Design review of the part built by this model. Coordinates are the model's own, in mm. A direction names the side the tool comes from. Give positions to 0.01 mm unless a question says otherwise; leave off trailing zeros. Write each loop counter-clockwise with the first axis right and the second up, starting at its lowest first coordinate (ties: lowest second). Pieces come first, ordered by that corner, then holes. Notation, with made-up numbers: (11, 12.5) - (63, 12.5) arc R14 ccw to (63, 36.5) - close; hole circle Ø5 at (81.25, -32). An arc over 180 degrees is marked (long way). Use a Markdown table: item, result. Add a question column.
```python
from build123d import *

# Parameters (mm, degrees)
F1_DEPTH = 2.1
F3_DEPTH = 1.8
F5_DEPTH = 8
F7_DEPTH = 1.016


with BuildPart() as f1:
    # F0 (on Top) → F1 (new body)
    with BuildSketch(Plane.XY):
        Polygon((61.593626, -18.5), (61.593626, 18.5), (-25.406374, 18.5), (-25.406374, 30.5), (-47.352125, 0), (-25.406374, -30.5), (-25.406374, -18.5), align=None)
    extrude(amount=F1_DEPTH)

    # F2 (on face) → F3 (join)
    with BuildSketch(Plane.XY.offset(2.1)):
        Polygon((59.493628, 16.400002), (-27.506373, 16.400002), (-27.506373, 23.985889), (-44.765007, 0), (-27.506373, -23.985889), (-27.506373, -16.400002), (59.493628, -16.400002), align=None)
        Polygon((-29.606375, 17.471772), (-29.606375, 14.3), (57.393626, 14.3), (57.393626, -14.3), (-29.606375, -14.3), (-29.606375, -17.471772), (-42.177888, 0), align=None, mode=Mode.SUBTRACT)
    extrude(amount=F3_DEPTH)

    # F4 (on face) → F5 (cut)
    with BuildSketch(Plane.XY.offset(2.1)):
        Polygon((-7.031372, -2.5), (-7.031372, 0), (-7.031372, 2.5), (-17.031372, 2.5), (-17.031372, -2.5), align=None)
    extrude(amount=-F5_DEPTH, mode=Mode.SUBTRACT)

    # F6 (on face) → F7 (cut)
    with BuildSketch(Plane(origin=(0, 0, 0), x_dir=(1, 0, 0), z_dir=(0, 0, -1))):
        with BuildLine():
            Line((17.868375, 5.807877), (17.389968, 6.649467))
            Line((17.389968, 6.649467), (15.720274, 6.649467))
            Line((15.720274, 6.649467), (11.672532, 6.649467))
            Line((11.672532, 6.649467), (10.458209, 7.054241))
            Line((10.458209, 7.054241), (9.49687, 7.459016))
            Line((9.49687, 7.459016), (8.484934, 7.914387))
            Line((8.484934, 7.914387), (7.776579, 8.369757))
            Line((7.776579, 8.369757), (6.461063, 8.369757))
            Line((6.461063, 8.369757), (6.461063, 7.054241))
            Line((6.461063, 7.054241), (6.865838, 5.688129))
            Line((6.865838, 5.688129), (7.827176, 4.524403))
            Line((7.827176, 4.524403), (8.484934, 3.411273))
            Line((8.484934, 3.411273), (8.484934, 1.437999))
            Line((8.484934, 1.437999), (9.49687, 0.881434))
            Line((9.49687, 0.881434), (9.49687, -1.749598))
            Line((9.49687, -1.749598), (10.002838, -2.710937))
            Line((10.002838, -2.710937), (10.458209, -3.621679))
            Line((10.458209, -3.621679), (10.458209, -6.050324))
            Line((10.458209, -6.050324), (11.014773, -6.505695))
            Line((11.014773, -6.505695), (11.672532, -6.505695))
            Line((11.672532, -6.505695), (12.077306, -6.100921))
            Line((12.077306, -6.100921), (12.532677, -6.100921))
            Line((12.532677, -6.100921), (12.90433, -6.582127))
            Line((12.90433, -6.582127), (13.527384, -6.100921))
            Line((13.527384, -6.100921), (14.296271, -7.096457))
            Line((14.296271, -7.096457), (15.720274, -7.096457))
            Line((15.720274, -7.096457), (16.735842, -7.573813))
            Line((16.735842, -7.573813), (17.14153, -8.114732))
            Line((17.14153, -8.114732), (17.637373, -8.790881))
            Line((17.637373, -8.790881), (17.637373, -10.098103))
            Line((17.637373, -10.098103), (18.358599, -10.729175))
            Line((18.358599, -10.729175), (18.944595, -10.729175))
            Line((18.944595, -10.729175), (19.39536, -11.134865))
            Line((19.39536, -11.134865), (21.333655, -11.134865))
            Line((21.333655, -11.134865), (22.505646, -10.684098))
            Line((22.505646, -10.684098), (22.862506, -10.359681))
            Line((22.862506, -10.359681), (26.547044, -10.359681))
            Line((26.547044, -10.359681), (27.159763, -9.794501))
            Line((27.159763, -9.794501), (29.251238, 6.794227))
            Line((29.251238, 6.794227), (31.42953, -10.359681))
            Line((31.42953, -10.359681), (34.922162, -10.359681))
            Line((34.922162, -10.359681), (34.922162, -9.405373))
            ThreePointArc((34.922162, -9.405373), (38.566072, -10.431832), (42.282903, -9.712898))
            ThreePointArc((42.282903, -9.712898), (43.887119, -8.50738), (45.256817, -7.040849))
            ThreePointArc((45.256817, -7.040849), (47.068037, -9.266569), (49.795189, -10.159309))
            ThreePointArc((49.795189, -10.159309), (52.782739, -8.771872), (54.433858, -5.921566))
            ThreePointArc((54.433858, -5.921566), (55.612943, 0.923855), (54.802926, 7.822689))
            ThreePointArc((54.802926, 7.822689), (53.159635, 11.066769), (49.981279, 12.833834))
            ThreePointArc((49.981279, 12.833834), (48.205281, 12.681465), (46.748952, 11.653607))
            ThreePointArc((46.748952, 11.653607), (42.496265, 12.988448), (38.243578, 11.653607))
            Line((38.243578, 11.653607), (38.243578, 12.988448))
            Line((38.243578, 12.988448), (34.899586, 12.988448))
            Line((34.899586, 12.988448), (33.07669, -4.188973))
            Line((33.07669, -4.188973), (31.098974, 12.775832))
            Line((31.098974, 12.775832), (27.543157, 12.775832))
            Line((27.543157, 12.775832), (25.559743, -4.294449))
            Line((25.559743, -4.294449), (23.376931, 12.895053))
            Line((23.376931, 12.895053), (17.104378, 12.895053))
            Line((17.104378, 12.895053), (18.728114, 11.108903))
            Line((18.728114, 11.108903), (18.844541, 10.192047))
            Line((18.844541, 10.192047), (19.452574, 10.054762))
            Line((19.452574, 10.054762), (19.452574, 9.066838))
            Line((19.452574, 9.066838), (19.316775, 8.465384))
            Line((19.316775, 8.465384), (19.452574, 8.434722))
            Line((19.452574, 8.434722), (19.570415, 7.506735))
            Line((19.570415, 7.506735), (20.018297, 7.40561))
            Line((20.018297, 7.40561), (20.151291, 6.358286))
            Line((20.151291, 6.358286), (20.264299, 6.33277))
            Line((20.264299, 6.33277), (19.990926, 5.122006))
            Line((19.990926, 5.122006), (20.075682, 4.454563))
            Line((20.075682, 4.454563), (19.6355, 3.658812))
            Line((19.6355, 3.658812), (19.6355, 2.990214))
            Line((19.6355, 2.990214), (20.065341, 1.93956))
            Line((20.065341, 1.93956), (20.065341, 1.223204))
            Line((20.065341, 1.223204), (19.73102, 0.697878))
            Line((19.73102, 0.697878), (19.062379, 0.697878))
            Line((19.062379, 0.697878), (18.680296, 0.077037))
            Line((18.680296, 0.077037), (17.725095, -0.687076))
            Line((17.725095, -0.687076), (16.722131, -0.687076))
            Line((16.722131, -0.687076), (16.398085, -0.327953))
            Line((16.398085, -0.327953), (16.00573, 0.124794))
            Line((16.00573, 0.124794), (16.722131, 0.745635))
            Line((16.722131, 0.745635), (17.389968, 0.745635))
            Line((17.389968, 0.745635), (18.154935, 1.748532))
            Line((18.154935, 1.748532), (19.014617, 1.748532))
            Line((19.014617, 1.748532), (19.014617, 2.464886))
            Line((19.014617, 2.464886), (18.680296, 2.990214))
            Line((18.680296, 2.990214), (18.680296, 3.658812))
            Line((18.680296, 3.658812), (19.205659, 4.088624))
            Line((19.205659, 4.088624), (19.205659, 4.94825))
            Line((19.205659, 4.94825), (18.728056, 4.94825))
            Line((18.728056, 4.94825), (18.298216, 4.375167))
            Line((18.298216, 4.375167), (17.725095, 3.658812))
            Line((17.725095, 3.658812), (17.389968, 3.181241))
            Line((17.389968, 3.181241), (16.722131, 3.181241))
            Line((16.722131, 3.181241), (16.722131, 3.658812))
            Line((16.722131, 3.658812), (17.389968, 4.136382))
            Line((17.389968, 4.136382), (17.389968, 4.900494))
            Line((17.389968, 4.900494), (17.868375, 4.900494))
            Line((17.868375, 4.900494), (17.868375, 5.807877))
        make_face()
        with BuildLine():
            Line((36.25592, -5.079472), (37.317255, 3.487003))
            Line((37.317255, 3.487003), (38.226967, 1.819194))
            Line((38.226967, 1.819194), (40.577063, -0.379282))
            Line((40.577063, -0.379282), (41.562585, -1.199999))
            Line((41.562585, -1.199999), (42.093252, -2.27452))
            ThreePointArc((42.093252, -2.27452), (42.411611, -3.810418), (41.941633, -5.3069))
            ThreePointArc((41.941633, -5.3069), (40.261644, -6.627542), (38.151158, -6.292424))
            Line((38.151158, -6.292424), (36.25592, -5.079472))
        make_face(mode=Mode.SUBTRACT)
        with BuildLine():
            Line((43.431631, 9.066838), (44.995993, 8.465384))
            Line((44.995993, 8.465384), (44.810452, 7.643624))
            Line((44.810452, 7.643624), (43.853124, 2.68892))
            Line((43.853124, 2.68892), (41.205642, 5.095722))
            ThreePointArc((41.205642, 5.095722), (40.786126, 5.667855), (40.622921, 6.358286))
            ThreePointArc((40.622921, 6.358286), (40.666306, 7.396519), (41.205642, 8.284735))
            ThreePointArc((41.205642, 8.284735), (42.217155, 8.964619), (43.431631, 9.066838))
        make_face(mode=Mode.SUBTRACT)
        with BuildLine():
            add(Edge.make_bspline(
                [(50.053255, 8.283923), (45.320541, 8.283923), (47.686898, -2.756179), (50.053255, -13.79628), (52.419612, -2.756179), (54.78597, 8.283923), (50.053255, 8.283923)],
                knots=[0, 0, 0, 2.094395, 2.094395, 4.18879, 4.18879, 6.283185, 6.283185, 6.283185], degree=2, weights=[1, 0.5, 1, 0.5, 1, 0.5, 1]))
        make_face(mode=Mode.SUBTRACT)
    extrude(amount=-F7_DEPTH, mode=Mode.SUBTRACT)


solid = f1.part
```
(1) Add section B-B (x = -39). State the section outline as (y, z) points.
(2) Add section C-C (y = -20). State the section outline as (x, z) points.
(3) For line 1 along Y through (x, z) = (10.5, 2.8); line 2 along Y through (x, z) = (-15.5, 0.45); line 3 along Z through (x, y) = (36, -17.5), list the stretches that pass through material, from the lowest coordinate up.
(4) Tool access review of faces 4 (the face through (26.565, -4.36, 0.501)), 5 (the face through (-36.257, -11.825, 2.987)), 6 (the face through (-25.406, -25, 1)), 7 (the face through (-7.031, 0, 1)), 8 (the face through (-35.804, -8.858, 2.987)): name each direction out of +Z, -Z, +X, -X, +Y, -Y from which nothing blocks a thin tool from reaching the whole face with its end or side.
(5) Add section A-A (z = 3.2). State the section outline as (x, y) points (3 decimals).
(6) Insertion check: pin 1 (1 mm diameter, centred on y = 13.5, z = 2, fed in from -X); pin 2 (0.5 mm diameter, centred on y = -1, z = 3, fed in from +X); pin 3 (0.8 mm diameter, centred on x = 17, z = 0.5, fed in from +Y); pin 4 (5 mm diameter, centred on x = 10, y = 12.5, fed in from +Z). Each pin has a flat end and moves straight along its axis. Give the tip position at first contact, or say it passes through.
(7) Mouldability with a two-part tool opening along X and no side actions: class faces 1 (the face through (-36.015, 12.161, 2.987)), 2 (the face through (39.386, -0.735, 0.501)), 3 (the face through (-6, 0, 0)) as +X half, -X half, draft (parallel to the pull), parting line (faces both ways), or undercut.
Answers follow:
| question | item | result |
|---|---|---|
| 1 | outline | (-11.61, 0) - (11.61, 0) - (11.61, 2.1) - (8.01, 2.1) - (8.01, 3.9) - (4.42, 3.9) - (4.42, 2.1) - (-4.42, 2.1) - (-4.42, 3.9) - (-8.01, 3.9) - (-8.01, 2.1) - (-11.61, 2.1) - close |
| 2 | outline | (-32.96, 0) - (-25.41, 0) - (-25.41, 2.1) - (-27.51, 2.1) - (-27.51, 3.9) - (-30.37, 3.9) - (-30.37, 2.1) - (-32.96, 2.1) - close |
| 3 | line 1 | -16.4 to -14.3, 14.3 to 16.4 |
| 3 | line 2 | -18.5 to -2.5, 2.5 to 18.5 |
| 3 | line 3 | 0 to 2.1 |
| 4 | face 4 | -Z |
| 4 | face 5 | +Z, -X, -Y |
| 4 | face 6 | +Z, -Z, +X, -Y |
| 4 | face 7 | +Z, -Z |
| 4 | face 8 | +Z |
| 5 | outline | (-44.765, 0) - (-27.506, -23.986) - (-27.506, -16.4) - (59.494, -16.4) - (59.494, 16.4) - (-27.506, 16.4) - (-27.506, 23.986) - close; hole (-42.178, 0) - (-29.606, -17.472) - (-29.606, -14.3) - (57.394, -14.3) - (57.394, 14.3) - (-29.606, 14.3) - (-29.606, 17.472) - close |
| 6 | pin 1 | x = -38 |
| 6 | pin 2 | x = 59.49 |
| 6 | pin 3 | y = 18.5 |
| 6 | pin 4 | z = 3.9 |
| 7 | face 1 | -X half |
| 7 | face 2 | undercut |
| 7 | face 3 | draft |
